Autodesk Inventor part; units mm, degrees
ref_plane "YZ Plane" through (0, 0, 0) normal (1, 0, 0) x (0, 1, 0)
ref_plane "XZ Plane" through (0, 0, 0) normal (0, 1, 0) x (-1, 0, 0)
ref_plane "XY Plane" through (0, 0, 0) normal (0, 0, 1) x (1, 0, 0)
ref_plane "Work Plane6" through (-21.8665, 24.3353, 26.2725) normal (0, 1, 0) x (-1, 0, 0)
sketch "Sketch1" plane through (-21.8665, 24.3353, 26.2725) normal (0, 1, 0) x (-1, 0, 0)
  line L0 (7.495, -2.8448) -> (7.8208, -2.519)
  line L1 (7.8208, -2.519) -> (7.8323, -2.5175)
  line L2 (7.8323, -2.5175) -> (8.2313, -2.7479)
  line L3 (8.2313, -2.7479) -> (8.4616, -2.3489)
  line L4 (8.4616, -2.3489) -> (8.4724, -2.3444)
  line L5 (8.4724, -2.3444) -> (8.9174, -2.4637)
  line L6 (8.9174, -2.4637) -> (9.0366, -2.0186)
  line L7 (9.0366, -2.0186) -> (9.0459, -2.0116)
  line L8 (9.0459, -2.0116) -> (9.5066, -2.0116)
  line L9 (9.5066, -2.0116) -> (9.5066, -1.5509)
  line L10 (9.5066, -1.5509) -> (9.5136, -1.5416)
  line L11 (9.5136, -1.5416) -> (9.9587, -1.4224)
  line L12 (9.9587, -1.4224) -> (9.8394, -0.9774)
  line L13 (9.8394, -0.9774) -> (9.8439, -0.9666)
  line L14 (9.8439, -0.9666) -> (10.2429, -0.7363)
  line L15 (10.2429, -0.7363) -> (10.0125, -0.3373)
  line L16 (10.0125, -0.3373) -> (10.014, -0.3258)
  line L17 (10.014, -0.3258) -> (10.3398, 0)
  line L18 (10.3398, 0) -> (10.014, 0.3258)
  line L19 (10.014, 0.3258) -> (10.0125, 0.3373)
  line L20 (10.0125, 0.3373) -> (10.2429, 0.7363)
  line L21 (10.2429, 0.7363) -> (9.8439, 0.9666)
  line L22 (9.8439, 0.9666) -> (9.8394, 0.9774)
  line L23 (9.8394, 0.9774) -> (9.9587, 1.4224)
  line L24 (9.9587, 1.4224) -> (9.5136, 1.5416)
  line L25 (9.5136, 1.5416) -> (9.5066, 1.5509)
  line L26 (9.5066, 1.5509) -> (9.5066, 2.0116)
  line L27 (9.5066, 2.0116) -> (9.0459, 2.0116)
  line L28 (9.0459, 2.0116) -> (9.0366, 2.0186)
  line L29 (9.0366, 2.0186) -> (8.9174, 2.4637)
  line L30 (8.9174, 2.4637) -> (8.4724, 2.3444)
  line L31 (8.4724, 2.3444) -> (8.4616, 2.3489)
  line L32 (8.4616, 2.3489) -> (8.2313, 2.7479)
  line L33 (8.2313, 2.7479) -> (7.8323, 2.5175)
  line L34 (7.8323, 2.5175) -> (7.8208, 2.519)
  line L35 (7.8208, 2.519) -> (7.495, 2.8448)
  line L36 (7.495, 2.8448) -> (7.1692, 2.519)
  line L37 (7.1692, 2.519) -> (7.1577, 2.5175)
  line L38 (7.1577, 2.5175) -> (6.7587, 2.7479)
  line L39 (6.7587, 2.7479) -> (6.5284, 2.3489)
  line L40 (6.5284, 2.3489) -> (6.5176, 2.3444)
  line L41 (6.5176, 2.3444) -> (6.0726, 2.4637)
  line L42 (6.0726, 2.4637) -> (5.9534, 2.0186)
  line L43 (5.9534, 2.0186) -> (5.9441, 2.0116)
  line L44 (5.9441, 2.0116) -> (5.4834, 2.0116)
  line L45 (5.4834, 2.0116) -> (5.4834, 1.5509)
  line L46 (5.4834, 1.5509) -> (5.4764, 1.5416)
  line L47 (5.4764, 1.5416) -> (5.0313, 1.4224)
  line L48 (5.0313, 1.4224) -> (5.1506, 0.9774)
  line L49 (5.1506, 0.9774) -> (5.1461, 0.9666)
  line L50 (5.1461, 0.9666) -> (4.7471, 0.7363)
  line L51 (4.7471, 0.7363) -> (4.9775, 0.3373)
  line L52 (4.9775, 0.3373) -> (4.976, 0.3258)
  line L53 (4.976, 0.3258) -> (4.6502, 0)
  line L54 (4.6502, 0) -> (4.976, -0.3258)
  line L55 (4.976, -0.3258) -> (4.9775, -0.3373)
  line L56 (4.9775, -0.3373) -> (4.7471, -0.7363)
  line L57 (4.7471, -0.7363) -> (5.1461, -0.9666)
  line L58 (5.1461, -0.9666) -> (5.1506, -0.9774)
  line L59 (5.1506, -0.9774) -> (5.0313, -1.4224)
  line L60 (5.0313, -1.4224) -> (5.4764, -1.5416)
  line L61 (5.4764, -1.5416) -> (5.4834, -1.5509)
  line L62 (5.4834, -1.5509) -> (5.4834, -2.0116)
  line L63 (5.4834, -2.0116) -> (5.9441, -2.0116)
  line L64 (5.9441, -2.0116) -> (5.9534, -2.0186)
  line L65 (5.9534, -2.0186) -> (6.0726, -2.4637)
  line L66 (6.0726, -2.4637) -> (6.5176, -2.3444)
  line L67 (6.5176, -2.3444) -> (6.5284, -2.3489)
  line L68 (6.5284, -2.3489) -> (6.7587, -2.7479)
  line L69 (6.7587, -2.7479) -> (7.1577, -2.5175)
  line L70 (7.1577, -2.5175) -> (7.1692, -2.519)
  line L71 (7.1692, -2.519) -> (7.495, -2.8448)
  circle A0 centre (7.495, 0) radius 1.25
  point P0 (-21.8665, -26.2725)
extrude "Extrusion1" add sketch "Sketch1" along normal blind 3
ref_plane "Work Plane5" through (-21.8665, 27.3353, 26.2725) normal (0, 1, 0) x (1, 0, 0)
sketch "Sketch4" plane through (-21.8665, 27.3353, 26.2725) normal (0, 1, 0) x (1, 0, 0)
  circle A0 centre (-7.495, 0) radius 1.25 construction
  circle A1 centre (-7.495, 0) radius 2.5
  point P0 (21.8665, 26.2725)
extrude "Extrusion2" add sketch "Sketch4" along normal blind 5
properties part number "servo_spine" material "Brass, Soft Yellow"
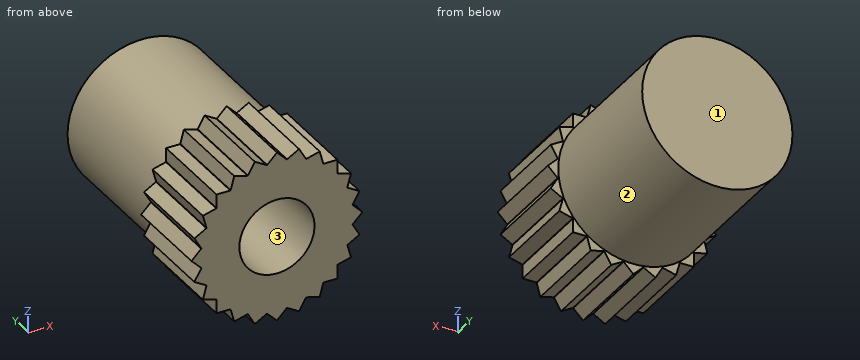
CAD build for the part. Positions are in the model's coordinates, mm. Face numbers are marked on the shaded views. Give positions to 0.01 mm unless a question says otherwise; leave off trailing zeros. Write each loop counter-clockwise with the first axis right and the second up, starting at its lowest first coordinate (ties: lowest second). Pieces come first, ordered by that corner, then holes. Notation, with made-up numbers: M -19,0.25 L 5,0.25 A15 cw 5,27.25 Z; hole C -28,4.5 d4. An arc over 180 degrees is marked long. Put each result on its own line as item: value. Start each with the question number.
(1) Band-saw the part on B-B, the plane y = 30. Write the cut outline in (x, z), and give its area (3 significant figures).
(2) Band-saw the part on D-D, the plane z = 26.4. Write the cut outline in (x, y), and give its area (3 significant figures).
(3) Band-saw the part on C-C, the plane x = -31.2. Write the cut outline in (y, z), and give its area (3 significant figures).
(4) Probe L1, parallel to X at y = 25.75, z = 26.65; L2, parallel to X at y = 31.25, z = 25.85; L3, parallel to Z at x = -29.45, y = 25.5. List the from-to ranges inside material, lowest first.
(5) Flat gauge pins, fed straight in: pin 1 Ø0.5 at (x, y) = (-31, 26) entering from +Z; pin 2 Ø0.5 at (x, y) = (-27.5, 26.5) entering from +Z; pin 3 Ø3 at (y, z) = (31.5, 24.5) entering from +X. Where does each tip first touch, or does it go through?
(6) Mould opens along X. For the marked faces 1, 2 and 3 say: +X half, -X half, draft (parallel to the pull), parting line (faces both ways), or undercut.
(7) Band-saw the part on A-A, the plane z = 24.6. Write the cut outline in (x, y), and give its area (3 significant figures).
Response values:
1. outline: C -29.36,26.27 d5
1. area: 19.6 mm2
2. outline: M -32.08,24.34 L -30.6,24.34 L -30.6,27.34 L -28.12,27.34 L -28.12,24.34 L -26.64,24.34 L -26.64,27.34 L -26.86,27.34 L -26.86,32.34 L -31.86,32.34 L -31.86,27.34 L -32.08,27.34 Z
2. area: 33.8 mm2
3. outline: M 24.34,24.26 L 27.34,24.26 L 27.34,24.58 L 32.34,24.58 L 32.34,27.97 L 27.34,27.97 L 27.34,28.28 L 24.34,28.28 Z
3. area: 29.0 mm2
4. L1: x = -31.9 to -30.55, -28.17 to -26.82
4. L2: x = -31.83 to -26.9
4. L3: z = 23.52 to 25.03, 27.52 to 29.03
5. pin 1: stops at z = 28.74
5. pin 2: stops at z = 28.28
5. pin 3: stops at x = -26.88
6. face 1: draft
6. face 2: parting line
6. face 3: undercut
7. outline: M -31.37,24.34 L -27.35,24.34 L -27.35,27.34 L -27.5,27.34 L -27.5,32.34 L -31.22,32.34 L -31.22,27.34 L -31.37,27.34 Z
7. area: 30.7 mm2
